Model file for the job. Use its own axes, mm. A direction names the side the tool comes from. Round coordinates to 2 decimals unless told otherwise and drop trailing zeros. Order: outer loops, then holes, each group sorted by start corner. A loop starts at its lowest first (then second) coordinate and runs counter-clockwise, first axis right, second up. Notation, with made-up numbers: (0, 85.25) - (59, 85.25) arc R8 cw to (59, 89.25) - close; hole circle Ø5 at (16.25, -36). An arc over 180 degrees is marked (long way). Write item = value, one per line.
```python
from build123d import *

# Parameters (mm, degrees)
SKETCH1_W           = 30
SKETCH1_H           = 45
SKETCH1_R           = 1.25
LASER_IF_DEPTH      = 3
SKETCH4_R           = 1
VLS_IF_TOP_DEPTH    = 4
SKETCH5_W           = 43
SKETCH5_H           = 20
SKETCH5_R           = 1
SKETCH5_W_2         = 18
SKETCH5_H_2         = 45
BOSS_EXTRUDE1_DEPTH = 3
FILLET1_R           = 10
FILLET2_R           = 5
BOSS_EXTRUDE2_DEPTH = 7
FILLET3_R           = 5
SKETCH7_W           = 18
SKETCH7_H           = 8
CUT_EXTRUDE1_DEPTH  = 83.182723245
FILLET4_R           = 10
FILLET5_R           = 10


with BuildPart() as part:
    # Sketch1 → LASER IF (new body)
    with BuildSketch(Plane(origin=(0, 22.5, 0), x_dir=(1, 0, 0), z_dir=(0, 1, 0))):
        with Locations((39, 16.5)):
            Rectangle(SKETCH1_W, SKETCH1_H)
        with Locations(Location((47, -3.75, 0), (0, 0, 270))):
            Circle(SKETCH1_R, mode=Mode.SUBTRACT)
        with Locations(Location((39, -3.75, 0), (0, 0, 270))):
            Circle(SKETCH1_R, mode=Mode.SUBTRACT)
        with Locations(Location((31, -3.75, 0), (0, 0, 270))):
            Circle(SKETCH1_R, mode=Mode.SUBTRACT)
        with Locations(Location((47, 36.75, 0), (0, 0, 270))):
            Circle(SKETCH1_R, mode=Mode.SUBTRACT)
        with Locations(Location((39, 36.75, 0), (0, 0, 270))):
            Circle(SKETCH1_R, mode=Mode.SUBTRACT)
        with Locations(Location((31, 36.75, 0), (0, 0, 270))):
            Circle(SKETCH1_R, mode=Mode.SUBTRACT)
    extrude(amount=LASER_IF_DEPTH)



with BuildPart() as body_2:
    # Sketch4 → VLS IF TOP (new body)
    with BuildSketch(Plane(origin=(0, 21.5, 0), x_dir=(1, 0, 0), z_dir=(0, 1, 0))):
        with BuildLine():
            Line((3.464101615, 12.5), (2.969229956, 9.071428571))
            ThreePointArc((2.969229956, 9.071428571), (0, 6.5), (-2.969229956, 9.071428571))
            Line((-2.969229956, 9.071428571), (-3.464101615, 12.5))
            ThreePointArc((-3.464101615, 12.5), (0, 16.5), (3.464101615, 12.5))
        make_face()
        with Locations(Location((0, 13, 0), (0, 0, 270))):
            Circle(SKETCH4_R, mode=Mode.SUBTRACT)
        with Locations(Location((0, 9.5, 0), (0, 0, 270))):
            Circle(SKETCH4_R, mode=Mode.SUBTRACT)
    extrude(amount=VLS_IF_TOP_DEPTH)


with BuildPart() as part_1:
    add(part.part)

    add(body_2.part)  # Boss-Extrude1 merges body 2
    # Sketch5 → Boss-Extrude1 (add)
    # profile 1 of 2: a face of its own
    with BuildSketch(Plane(origin=(0, 25.5, 0), x_dir=(1, 0, 0), z_dir=(0, 1, 0))):
        with Locations((2.5, 12)):
            Rectangle(SKETCH5_W, SKETCH5_H)
        with Locations(Location((0, 9.5, 0), (0, 0, 270))):
            Circle(SKETCH5_R, mode=Mode.SUBTRACT)
        with Locations(Location((0, 13, 0), (0, 0, 270))):
            Circle(SKETCH5_R, mode=Mode.SUBTRACT)
    # profile 2 of 2: a face of its own
    with BuildSketch(Plane(origin=(0, 25.5, 0), x_dir=(1, 0, 0), z_dir=(0, 1, 0))):
        with Locations((63, 16.5)):
            Rectangle(SKETCH5_W_2, SKETCH5_H_2)
    extrude(amount=-BOSS_EXTRUDE1_DEPTH)

    # Fillet1
    # the kernel refuses this fillet: 10 mm, written as the material it adds along each edge
    with BuildSketch(Plane(origin=(24, 25.5, -2), x_dir=(-1, 0, 0), z_dir=(0, -1, 0))) as fillet1_piece_1:
        with BuildLine():
            CenterArc((9.797958971, -10), FILLET1_R, 90, 78.463040967)
            Line((0, -8), (-0.195959179, -7.96))
            ThreePointArc((-0.195959179, -7.96), (-0.2, -4), (-0.2, 0))
            Line((-0.2, 0), (0, 0.2))
            Line((0, 0.2), (9.797958971, 0.2))
            Line((9.797958971, 0.2), (9.797958971, 0))
        make_face()
    extrude(amount=3)
    with BuildSketch(Plane(origin=(24, 25.5, -22), x_dir=(-1, 0, 0), z_dir=(0, -1, 0))) as fillet1_piece_2:
        with BuildLine():
            CenterArc((FILLET1_R, FILLET1_R), FILLET1_R, 180, 90)
            Line((0, FILLET1_R), (-FILLET1_R * 0.02, FILLET1_R))
            Line((-FILLET1_R * 0.02, FILLET1_R), (-FILLET1_R * 0.02, -FILLET1_R * 0.02))
            Line((-FILLET1_R * 0.02, -FILLET1_R * 0.02), (FILLET1_R, -FILLET1_R * 0.02))
            Line((FILLET1_R, -FILLET1_R * 0.02), (FILLET1_R, 0))
        make_face()
    extrude(amount=3)

    # Fillet2
    fillet2_edges = [part_1.edges().sort_by_distance(p)[0] for p in [
        (24, 24, -39),
        (24, 24, 6),
    ]]
    fillet(fillet2_edges, radius=FILLET2_R)

    # Sketch6 → Boss-Extrude2 (add)
    with BuildSketch(Plane(origin=(0, 25.5, 0), x_dir=(1, 0, 0), z_dir=(0, 1, 0))):
        Polygon((-16, 2), (-19, 2), (-19, 22), (69, 22), (69, 39), (72, 39), (72, 2), (69, 2), (69, 19), (-16, 19), align=None)
    extrude(amount=BOSS_EXTRUDE2_DEPTH)

    # Fillet3
    fillet3_edges = [part_1.edges().sort_by_distance(p)[0] for p in [
        (-16, 29, -19),
        (69, 29, -19),
        (69, 29, -22),
    ]]
    fillet(fillet3_edges, radius=FILLET3_R)

    # Sketch7 → Cut-Extrude1 (cut, through all)
    with BuildSketch(Plane(origin=(0, 25.5, 0), x_dir=(1, 0, 0), z_dir=(0, 1, 0))):
        with Locations((63, -2)):
            Rectangle(SKETCH7_W, SKETCH7_H)
    extrude(amount=-CUT_EXTRUDE1_DEPTH, mode=Mode.SUBTRACT)

    # Fillet4
    # the kernel refuses this fillet: 10 mm, written as the material it adds along each edge
    with BuildSketch(Plane(origin=(54, 25.5, -2), x_dir=(0, 0, 1), z_dir=(0, -1, 0))) as fillet4_piece_1:
        with BuildLine():
            CenterArc((10, -9.797958971), FILLET4_R, 101.536959033, 78.463040967)
            Line((0, -9.797958971), (-0.2, -9.797958971))
            Line((-0.2, -9.797958971), (-0.2, 0))
            Line((-0.2, 0), (0, 0.2))
            ThreePointArc((0, 0.2), (4, 0.2), (7.96, 0.195959179))
            Line((7.96, 0.195959179), (8, 0))
        make_face()
    extrude(amount=3)

    # Fillet5
    fillet5_edges = [part_1.edges().sort_by_distance(p)[0] for p in [
        (54, 24, 6),
    ]]
    fillet(fillet5_edges, radius=FILLET5_R)


solid = part_1.part
```
1) Flat gauge pins, fed straight in: pin 1 Ø3 at (x, z) = (39, -36.75) entering from -Y; pin 2 Ø3.5 at (x, y) = (10.5, 30) entering from +Z; pin 3 Ø8.5 at (x, z) = (44, -28) entering from +Y; pin 4 Ø2.5 at (x, z) = (0, -9.5) entering from -Y. Where does each tip first touch, or does it go through?
Conclusion:
pin_1 = 22.5
pin_2 = -19
pin_3 = 25.5
pin_4 = 21.5
2) Cut at B-B (y = 24). Give the number of separate pieces and of enclosed holes in the cut face, and give its area (3 significant figures).
Conclusion:
separate_pieces = 1
enclosed_holes = 8
area = 2,890 mm^2
3) Cut at A-A (x = 39). Write the cut outline in (y, z).
Conclusion:
outline = (22.5, -39) - (25.5, -39) - (25.5, -38) - (22.5, -38) - close; (22.5, -35.5) - (25.5, -35.5) - (25.5, -22) - (32.5, -22) - (32.5, -19) - (25.5, -19) - (25.5, 2.5) - (22.5, 2.5) - close; (22.5, 5) - (25.5, 5) - (25.5, 6) - (22.5, 6) - close
4) Cut at C-C (y = 31.25). Write the cut outline in (x, z).
Conclusion:
outline = (-19, -22) - (64, -22) arc R5 cw to (69, -27) - (69, -39) - (72, -39) - (72, -2) - (69, -2) - (69, -14) arc R5 cw to (64, -19) - (-11, -19) arc R5 cw to (-16, -14) - (-16, -2) - (-19, -2) - close
5) Cut at D-D (z = -36.75). Write the cut outline in (x, y), and give its area (3 significant figures).
Conclusion:
outline = (24.82, 22.5) - (29.75, 22.5) - (29.75, 25.5) - (24.82, 25.5) - close; (32.25, 22.5) - (37.75, 22.5) - (37.75, 25.5) - (32.25, 25.5) - close; (40.25, 22.5) - (45.75, 22.5) - (45.75, 25.5) - (40.25, 25.5) - close; (48.25, 22.5) - (72, 22.5) - (72, 32.5) - (69, 32.5) - (69, 25.5) - (48.25, 25.5) - close
area = 140 mm^2
6) 3-axis set-ups, long thin cutter, end or side, ignore diameter. For faces 1 (the face through (70, 26, -2)), 2 (the face through (-6, 25, -2)), 3 (the face through (-14, 29, -18)), 4 (the face through (39, 24, -38)): which of +Z, -Z, +X, -X, +Y, -Y reach the whole face in a straight line?
Conclusion:
face_1 = +Z, +X, +Y, -Y
face_2 = +Z, -X, +Y, -Y
face_3 = +Z, +Y
face_4 = +Y, -Y
7) Wall check: line 1 along X through (y, z) = (26.5, -7); line 2 along Y through (x, z) = (36, -4); line 3 along Z through (x, y) = (50.5, 26.25). Give the ranges that are in metal, low to high.
Conclusion:
line_1 = -19 to -16, 69 to 72
line_2 = 22.5 to 25.5
line_3 = -22 to -19
8) Mould opens along Z. For faces 5 (the face through (25, 24, -37)), 6 (the face through (0, 23, -12)), 7 (the face through (0, 21.5, -11.6)) say: +Z half, -Z half, draft (parallel to the pull), parting line (faces both ways), or undercut.
Conclusion:
face_5 = -Z half
face_6 = undercut
face_7 = draft
